from build123d import *

# Parameters (mm, degrees)
SKETCH1_W           = 100
SKETCH1_H           = 100
BOSS_EXTRUDE1_DEPTH = 3
BOSS_EXTRUDE2_DEPTH = 40
SKETCH3_R           = 5
CUT_EXTRUDE1_DEPTH  = 40


with BuildPart() as part:
    # Sketch1 → Boss-Extrude1 (new body)
    with BuildSketch(Plane.XY):
        with Locations((50, -50)):
            Rectangle(SKETCH1_W, SKETCH1_H)
    extrude(amount=BOSS_EXTRUDE1_DEPTH)

    # Sketch2 → Boss-Extrude2 (add)
    with BuildSketch(Plane.XY.offset(3)):
        Polygon((0, 0), (100, 0), (100, -5), (100, -100), (61, -100), (61, -95), (95, -95), (95, -5), (5, -5), (5, -95), (34, -95), (34, -100), (0, -100), (0, -6.075944417), align=None)
    extrude(amount=BOSS_EXTRUDE2_DEPTH)

    # Sketch3 → Cut-Extrude1 (cut)
    with BuildSketch(Plane.XZ.offset(100)):
        with Locations((75, 21.806521963)):
            Circle(SKETCH3_R)
    extrude(amount=-CUT_EXTRUDE1_DEPTH, mode=Mode.SUBTRACT)


solid = part.part
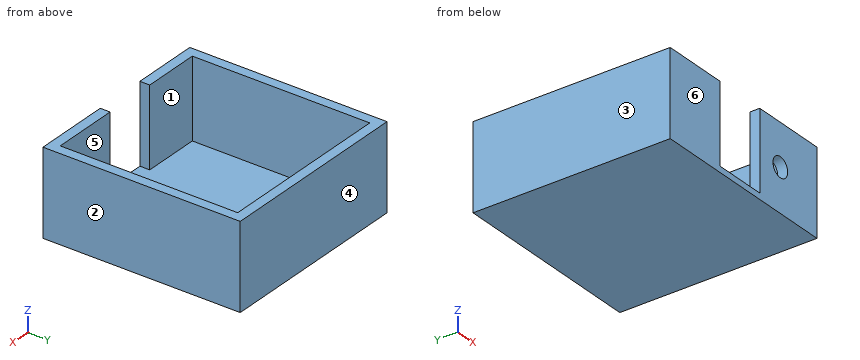
The model under review builds one solid part; all positions refer to its coordinate system, in mm. Face numbers are marked on the shaded views. A direction names the side the tool comes from. Give positions to 0.01 mm unless a question says otherwise; leave off trailing zeros. Write each loop counter-clockwise with the first axis right and the second up, starting at its lowest first coordinate (ties: lowest second). Pieces come first, ordered by that corner, then holes. Notation, with made-up numbers: M 78.5,32 L 115.5,32 A24 cw 115.5,54 Z; hole C 31.25,16.25 d1. An arc over 180 degrees is marked long. One line per question, with ' | ' between items. Start each with the question number.
Item 1: For the marked faces 5 and 6, list the 3-axis set-ups (+Z, -Z, +X, -X, +Y, -Y) from which the entire face can be reached by the end or side of a thin tool; tool diameter is ignored.
Item 2: Draft analysis for pull direction X (two halves, no side actions). For the marked faces 1, 2, 3 and 4, state which applies: released by +X, released by -X, zero draft, split by the parting line, or undercut.
Item 3: We need section D-D on x = 17. Write out the cut boundary in (y, z), plus the area to 3 significant figures.
Item 4: We need section B-B on y = -88.5. Write out the cut boundary in (x, z), plus the area to 3 significant figures.
Item 5: We need section C-C on z = 31.5. Write out the cut boundary in (x, y), plus the area to 4 significant figures.
Item 6: Wall thickness on line 1 (X direction, y = -75, z = 27); line 2 (Y direction, x = 21, z = 9); line 3 (Z direction, x = 75, y = -98.3): over which ranges is each line inside the solid? List them lowest first. Write a range as from..to.
Item 7: We need section A-A on x = 75. Write out the cut boundary in (y, z).
Results found:
1) face 5: +Z | face 6: +Z, -Z, +X, -X, -Y
2) face 1: undercut | face 2: released by +X | face 3: released by -X | face 4: zero draft
3) outline: M -100,0 L 0,0 L 0,43 L -5,43 L -5,3 L -95,3 L -95,43 L -100,43 Z | area: 700 mm2
4) outline: M 0,0 L 100,0 L 100,43 L 95,43 L 95,3 L 5,3 L 5,43 L 0,43 Z | area: 700 mm2
5) outline: M 0,-100 L 34,-100 L 34,-95 L 5,-95 L 5,-5 L 95,-5 L 95,-95 L 61,-95 L 61,-100 L 100,-100 L 100,0 L 0,0 Z | area: 1,765 mm2
6) line 1: x = 0..5, 95..100 | line 2: y = -100..-95, -5..0 | line 3: z = 0..16.81, 26.81..43
7) outline: M -100,0 L 0,0 L 0,43 L -5,43 L -5,3 L -95,3 L -95,16.81 L -100,16.81 Z; M -100,26.81 L -95,26.81 L -95,43 L -100,43 Z
